Check sheet for the drawn part. Datum: minimum x, y, z corner. Units: mm. Round coordinates to 2 decimals unless told otherwise and drop trailing zeros. Write each loop counter-clockwise with the first axis right and the second up, starting at its lowest first coordinate (ties: lowest second). Pieces come first, ordered by that corner, then holes.
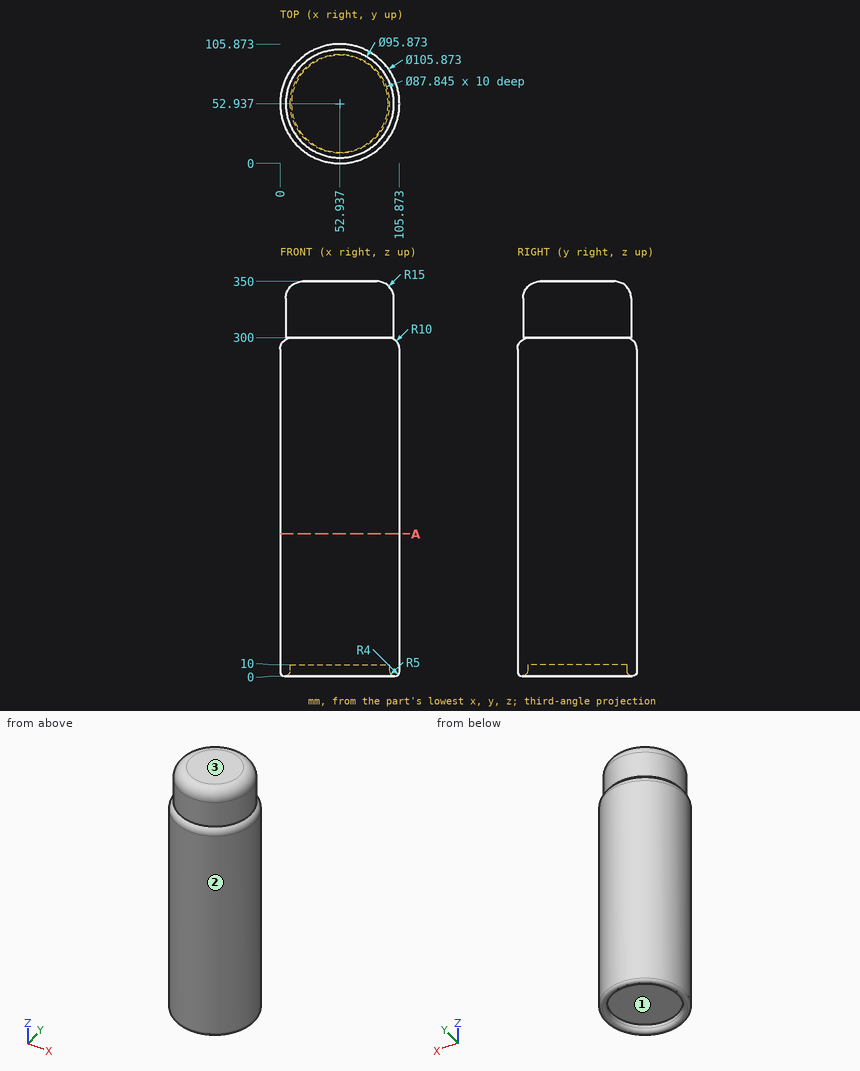
1. Sectioned sample at A-A, the plane z = 126. Enter the section's corners in (x, y).
2. Go/stop test with flat-tipped pins: pin 1 (3 mm diameter, centred on y = 62.5, z = 272, fed in from +X) (1 decimal); pin 2 (2 mm diameter, centred on x = 30.5, z = 285.5, fed in from -Y) (1 decimal); pin 3 (2 mm diameter, centred on x = 80, z = 280, fed in from +Y). Record where each tip stops, or that it passes through.
3. Scan lines: line 1 along Z through (x, y) = (55, 79); line 2 along Z through (x, y) = (97.5, 46.5) (1 decimal); line 3 along X through (y, z) = (52, 193.5) (1 decimal). Record each from-to range of solid material in increasing order.
4. Release check for a two-part mould opening along X. For the marked faces 1, 2 and 3 record: released by +X, released by -X, zero draft, split by the parting line, or undercut.
Computed values:
1. outline: circle Ø105.87 at (52.94, 52.94)
2. pin 1: stops at x = 105.3
2. pin 2: stops at y = 4.5
2. pin 3: stops at y = 99.01
3. line 1: z = 10 to 350
3. line 2: z = 1.9 to 299.8, 300 to 343.9
3. line 3: x = 0 to 105.9
4. face 1: undercut
4. face 2: split by the parting line
4. face 3: zero draft
